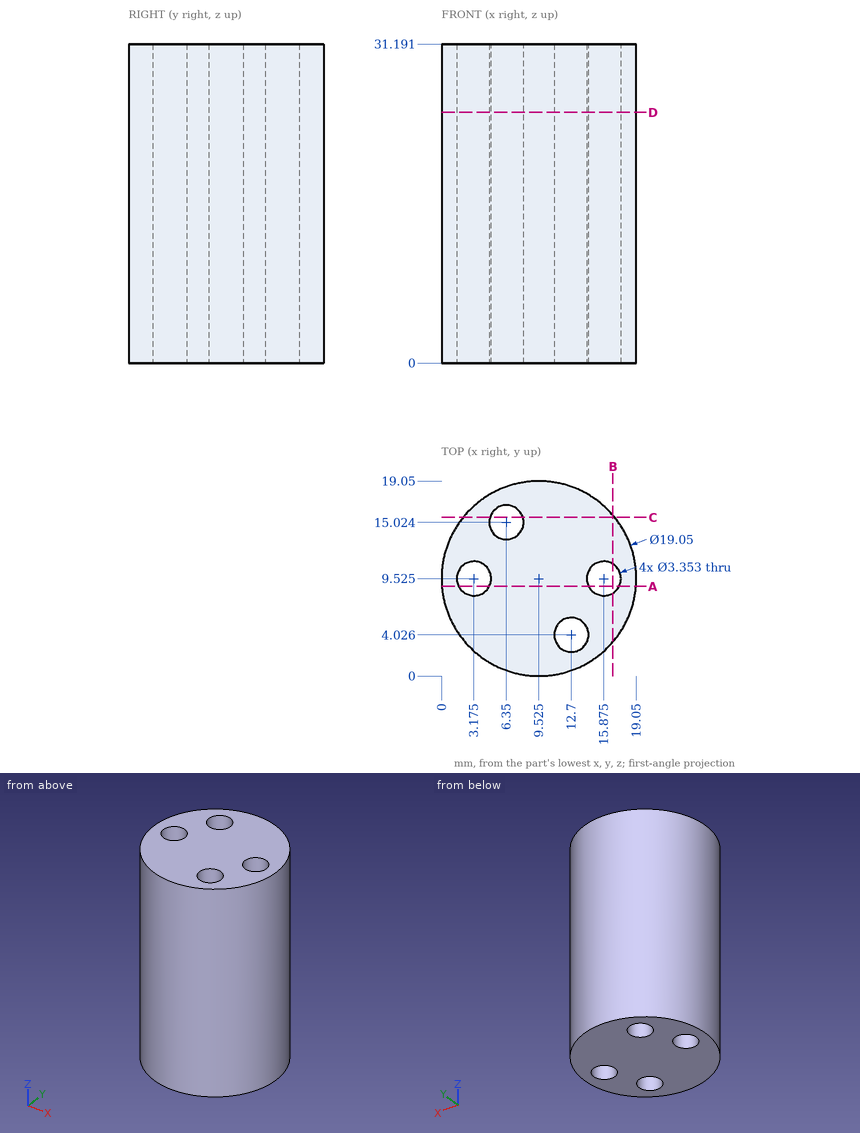
Geometry check sheet. Reference: drawing and pictorial views, mm from the part's lowest x, y, z. Give positions to 0.01 mm unless a question says otherwise; leave off trailing zeros. Order: outer loops, then holes, each group sorted by start corner. A loop starts at its lowest first (then second) coordinate and runs counter-clockwise, first axis right, second up.
1. Section check D-D, the plane z = 24.5. Give the number of separate pieces and of enclosed holes in the cut face, and give its area (3 significant figures).
2. Section check A-A, the plane y = 8.75. Enter the section's corners in (x, z).
3. Gauge pin test, flat ends, axial feed: pin 1 Ø2.5 at (x, y) = (15.875, 9.525) entering from -Z; pin 2 Ø1 at (y, z) = (5.5, 9.5) entering from -X; pin 3 Ø6 at (y, z) = (8, 18) entering from -X; pin 4 Ø3 at (y, z) = (16, 25) entering from -X. Record the tip position at first contact, or that the pin passes through.
4. Section check B-B, the plane x = 16.75. Enter the section's corners in (y, z) (1 decimal), and give its area (3 significant figures).
5. Thickness scan on L1, parallel to X at y = 9.25, z = 8.5; L2, parallel to X at y = 10.75, z = 19; L3, parallel to Y at x = 12.5, z = 26. Record the ranges inside material, lowest first.
6. Section check C-C, the plane y = 15.5. Enter the section's corners in (x, z).
Values follow:
1. separate pieces: 1
1. enclosed holes: 4
1. area: 250 mm2
2. outline: (0.03, 0) - (1.69, 0) - (1.69, 31.19) - (0.03, 31.19) - close; (4.66, 0) - (14.39, 0) - (14.39, 31.19) - (4.66, 31.19) - close; (17.36, 0) - (19.02, 0) - (19.02, 31.19) - (17.36, 31.19) - close
3. pin 1: passes through
3. pin 2: stops at x = 0.68
3. pin 3: stops at x = 0
3. pin 4: stops at x = 1.4
4. outline: (3.3, 0) - (8.1, 0) - (8.1, 31.2) - (3.3, 31.2) - close; (11, 0) - (15.7, 0) - (15.7, 31.2) - (11, 31.2) - close
4. area: 298 mm2
5. L1: x = 0 to 1.52, 4.83 to 14.22, 17.53 to 19.05
5. L2: x = 0.08 to 2.03, 4.32 to 14.73, 17.02 to 18.97
5. L3: y = 0.48 to 2.36, 5.69 to 18.57
6. outline: (2.11, 0) - (4.74, 0) - (4.74, 31.19) - (2.11, 31.19) - close; (7.96, 0) - (16.94, 0) - (16.94, 31.19) - (7.96, 31.19) - close
